```python
from build123d import *

# Parameters (mm, degrees)
F0_W     = 40
F0_H     = 80
F0_W_2   = 32
F0_H_2   = 72
F1_DEPTH = 200
F2_R     = 10.1
F3_DEPTH = 40.001
F4_R     = 2.5
F5_DEPTH = 40.001


with BuildPart() as f1:
    # F0 (on Front) → F1 (new body)
    with BuildSketch(Plane.XZ):
        Rectangle(F0_W, F0_H)
        Rectangle(F0_W_2, F0_H_2, mode=Mode.SUBTRACT)
    extrude(amount=F1_DEPTH)

    # F2 (on face) → F3 (cut, through all)
    with BuildSketch(Plane.YZ.offset(20)):
        with Locations((-100, 0)):
            Circle(F2_R)
    extrude(amount=-F3_DEPTH, mode=Mode.SUBTRACT)

    # F4 (on face) → F5 (cut, through all)
    with BuildSketch(Plane.YZ.offset(20)):
        with Locations((-125.547749, -14.75)):
            Circle(F4_R)
        with Locations((-125.547749, 14.75)):
            Circle(F4_R)
        with Locations((-100, 29.5)):
            Circle(F4_R)
        with Locations((-74.452251, 14.75)):
            Circle(F4_R)
        with Locations((-74.452251, -14.75)):
            Circle(F4_R)
        with Locations((-100, -29.5)):
            Circle(F4_R)
    extrude(amount=-F5_DEPTH, mode=Mode.SUBTRACT)


solid = f1.part
```
The model under review builds one solid part; all positions refer to its coordinate system, in mm. A direction names the side the tool comes from. Round coordinates to 2 decimals unless told otherwise and drop trailing zeros. Order: outer loops, then holes, each group sorted by start corner. A loop starts at its lowest first (then second) coordinate and runs counter-clockwise, first axis right, second up.
(1) Mouldability with a two-part tool opening along Z and no side actions: class faces 3 (the face through (18.03, -98.66, -27.39)), 4 (the face through (-16.4, -200, 3.1)), 5 (the face through (0, -99, -40)) as released by +Z, released by -Z, zero draft, split by the parting line, or undercut.
Working result:
face 3: undercut
face 4: zero draft
face 5: released by -Z
(2) For P1, Ø3, axis at y = -100, z = 29.5, coming from the +X side; P2, Ø6, axis at y = -125.55, z = -14.75, coming from the -X side, all flat-tipped, find the tip position at first contact; note any pin that passes through.
Working result:
P1: passes through
P2: stops at x = -20
(3) Take a section at C-C, the plane z = 29.5. State the section outline as (x, y) points.
Working result:
outline: (-20, -200) - (-16, -200) - (-16, -102.5) - (-20, -102.5) - close; (-20, -97.5) - (-16, -97.5) - (-16, 0) - (-20, 0) - close; (16, -200) - (20, -200) - (20, -102.5) - (16, -102.5) - close; (16, -97.5) - (20, -97.5) - (20, 0) - (16, 0) - close
(4) Take a section at A-A, the plane z = 14.75. State the section outline as (x, y) points.
Working result:
outline: (-20, -200) - (-16, -200) - (-16, -128.05) - (-20, -128.05) - close; (-20, -123.05) - (-16, -123.05) - (-16, -76.95) - (-20, -76.95) - close; (-20, -71.95) - (-16, -71.95) - (-16, 0) - (-20, 0) - close; (16, -200) - (20, -200) - (20, -128.05) - (16, -128.05) - close; (16, -123.05) - (20, -123.05) - (20, -76.95) - (16, -76.95) - close; (16, -71.95) - (20, -71.95) - (20, 0) - (16, 0) - close
(5) Tool access review of faces 1 (the face through (16, -99, -17)), 2 (the face through (18.028, -124.394, -16.968)): name each direction out of +Z, -Z, +X, -X, +Y, -Y from which nothing blocks a thin tool from reaching the whole face with its end or side.
Working result:
face 1: +Y, -Y
face 2: +X, -X
(6) Take a section at D-D, the plane y = -100. Count the separate pieces of the cut face and the enclosed holes in it, plus the area to 3 significant figures.
Working result:
separate pieces: 6
enclosed holes: 0
area: 654 mm2
(7) Take a section at B-B, the plane y = -133. State the section outline as (x, z) points, plus the area to 3 significant figures.
Working result:
outline: (-20, -40) - (20, -40) - (20, 40) - (-20, 40) - close; hole (-16, -36) - (16, -36) - (16, 36) - (-16, 36) - close
area: 896 mm2
(8) Wall thickness on L1, parallel to Z at x = 17.95, y = -100; L2, parallel to Z at x = 4, y = -54; L3, parallel to X at y = -116, z = 18: over which ranges is each line inside the solid? List them lowest first.
Working result:
L1: z = -40 to -32, -27 to -10.1, 10.1 to 27, 32 to 40
L2: z = -40 to -36, 36 to 40
L3: x = -20 to -16, 16 to 20
